Autodesk Inventor part; units mm, degrees
ref_plane "YZ Plane" through (0, 0, 0) normal (1, 0, 0) x (0, 1, 0)
ref_plane "XZ Plane" through (0, 0, 0) normal (0, 1, 0) x (-1, 0, 0)
ref_plane "XY Plane" through (0, 0, 0) normal (0, 0, 1) x (1, 0, 0)
sketch "Sketch1" plane through (0, 0, 0) normal (0, 1, 0) x (-1, 0, 0)
  line L0 (12.8, 0) -> (12.8, 32.2)
  line L1 (12.8, 16.1) -> (0, 16.1)
  line L2 (0, 0) -> (0, 32.2)
  line L3 (6.4, 27.2) -> (12.3, 27.2)
  line L4 (12.3, 27.2) -> (12.3, 5)
  line L5 (12.3, 5) -> (0.5, 5)
  line L6 (0.5, 5) -> (0.5, 27.2)
  line L7 (0.5, 27.2) -> (6.4, 27.2)
  line L8 (0, 0) -> (12.8, 0)
  circle A0 centre (6.4, 2.5) radius 0.5
  line L9 (0, 32.2) -> (12.8, 32.2)
  circle A1 centre (6.4, 29.7) radius 0.5
  line L10 (12.8, 32.2) -> (15.8, 32.2)
  line L11 (15.8, 32.2) -> (15.8, 0)
  line L12 (15.8, 0) -> (12.8, 0)
  line L13 (12.8, 0) -> (12.8, 32.2)
  point P0 (0, 0)
  dimension "d0" = 5.9
  dimension "d1" = 11.8
  dimension "d2" = 1
  dimension "d3" = 1
  dimension "d4" = 3
extrude "Extrusion1" add sketch "Sketch1" along normal blind 3 contours L8 L2 L1 L6 L5 L4 L0 | L0 L10 L11 L12 | L1 L4 L3 L7 L6 L2 L9 L0
sketch "Sketch2" plane through (0, 3, 0) normal (0, 1, 0) x (1, 0, 0)
  line L0 (-15.8, 0) -> (-15.8, -32.2)
  line L1 (0, 0) -> (-15.8, 0)
  line L2 (-15.8, -32.2) -> (-12.3, -32.2)
  line L3 (-12.3, -32.2) -> (-12.3, 0)
  line L4 (-12.3, 0) -> (-15.8, 0)
  line L5 (-15.8, 0) -> (-15.8, -32.2)
  dimension "d7" = 3.5
extrude "Extrusion2" add sketch "Sketch2" along normal blind 13
fillet "Fillet1" radius 2 1 edges at (-15.8, 0, 16.1)
sketch "Sketch3" plane through (-15.8, 16, 0) normal (-1, 0, 0) x (0, 0, 1)
  line L0 (32.2, -14) -> (32.2, 0)
  line L1 (32.2, -14) -> (0, -14)
  line L2 (32.2, 0) -> (51.999, 0) construction
  circle A0 centre (25.2, -7) radius 1.35
  line L3 (25.2, -7) -> (32.7, -7) construction
  circle A1 centre (17.7, -7) radius 0.65
  circle A2 centre (15.2, -7) radius 0.65
  circle A3 centre (12.7, -7) radius 0.65
  point P0 (0, -16)
  dimension "d12" = 2.7
  dimension "d17" = 1.3
  dimension "d18" = 1.3
  dimension "d19" = 1.3
extrude "Extrusion3" cut sketch "Sketch3" against normal blind 13
fillet "Fillet2" radius 2 4 edges at (-14.05, 16, 0) (-14.05, 16, 32.2) (0, 1.5, 32.2) (0, 1.5, 0)
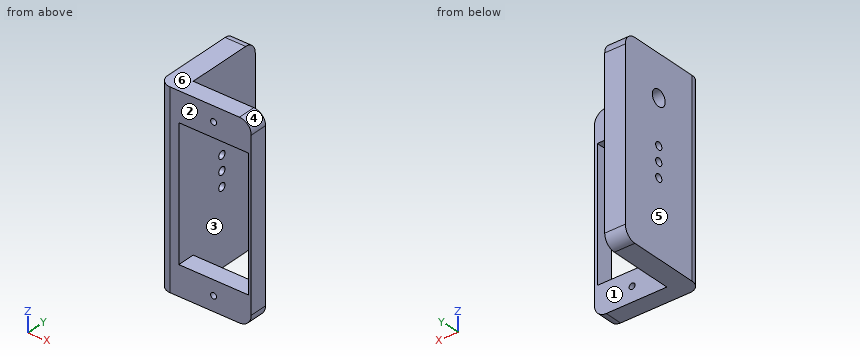
Geometry: final body of the model. Coordinates: model frame, mm. Face numbers are marked on the shaded views. A direction names the side the tool comes from. Give positions to 0.01 mm unless a question says otherwise; leave off trailing zeros. Loops run counter-clockwise (first coordinate to the right, second up) from the corner with the lowest first, then second, coordinate; pieces in that order, holes last. Notation, with made-up numbers: (-37, -33.75) -> (-1, -33.75) arc R27 cw to (-1, -14.75) -> close; hole circle Ø3 at (-0.75, 57). An arc over 180 degrees is marked (long way). Return JSON: item names as keys, results as strings.
Item 1: Mould query, pull axis X, two halves, no side actions, for the marked faces 3, 4, 5 and 6. Classes: released by +X, released by -X, zero draft, split by the parting line, or undercut.
Filled in:
{"face 3": "undercut", "face 4": "released by +X", "face 5": "released by -X", "face 6": "zero draft"}
Item 2: Pin query (flat end, axial travel): P1, Ø1.7, axis at y = 9, z = 17.7, coming from the +X side; P2, Ø6, axis at x = -11, z = 23.5, coming from the -Y side. Return the tip coordinate at first contact, or that it passes through.
Filled in:
{"P1": "x = -12.3", "P2": "y = 0"}
Item 3: Section D-D, the plane z = 29.7. Output: boundary loops of the cut face in (x, y).
Filled in:
{"outline": "(-15.8, 2) arc R2 ccw to (-13.8, 0) -> (-6.9, 0) -> (-6.9, 3) -> (-12.3, 3) -> (-12.3, 16) -> (-15.8, 16) -> close; (-5.9, 0) -> (0, 0) -> (0, 3) -> (-5.9, 3) -> close"}
Item 4: Section B-B, the plane z = 25.2. Output: boundary loops of the cut face in (x, y).
Filled in:
{"outline": "(-15.8, 2) arc R2 ccw to (-13.8, 0) -> (-12.3, 0) -> (-12.3, 7.65) -> (-15.8, 7.65) -> close; (-15.8, 10.35) -> (-12.3, 10.35) -> (-12.3, 16) -> (-15.8, 16) -> close; (-0.5, 0) -> (0, 0) -> (0, 3) -> (-0.5, 3) -> close"}
Item 5: Line query: line 1 (Y direction, x = -13.8, z = 25.2); line 2 (Z direction, x = -6.4, y = 0.75); line 3 (Z direction, x = -12.5, y = 8.5). Output: solid intervals per line, ascending.
Filled in:
{"line 1": "0 to 7.65, 10.35 to 16", "line 2": "0 to 2, 3 to 5, 27.2 to 29.2, 30.2 to 32.2", "line 3": "0 to 12.28, 13.12 to 14.78, 15.62 to 17.28, 18.12 to 23.95, 26.45 to 32.2"}
Item 6: Section C-C, the plane x = -12.75. Output: boundary loops of the cut face in (y, z).
Filled in:
{"outline": "(0, 0) -> (14, 0) arc R2 ccw to (16, 2) -> (16, 30.2) arc R2 ccw to (14, 32.2) -> (0, 32.2) -> close; hole circle Ø2.7 at (9, 25.2); hole circle Ø1.3 at (9, 12.7); hole circle Ø1.3 at (9, 15.2); hole circle Ø1.3 at (9, 17.7)"}
Item 7: Access query for the marked faces 1 and 2. Directions: +Z, -Z, +X, -X, +Y, -Y. A direction counts if a zero-diameter tool reaches every point of the face in a straight line with its end or side. Return the directions, or none.
Filled in:
{"face 1": "+Z, -Z, +X, +Y", "face 2": "+Z, -Z, +X, -X, -Y"}
Item 8: Section A-A, the plane x = -6.4. Output: boundary loops of the cut face in (y, z), plus the area to 3 significant figures.
Filled in:
{"outline": "(0, 0) -> (3, 0) -> (3, 2) -> (0, 2) -> close; (0, 3) -> (3, 3) -> (3, 5) -> (0, 5) -> close; (0, 27.2) -> (3, 27.2) -> (3, 29.2) -> (0, 29.2) -> close; (0, 30.2) -> (3, 30.2) -> (3, 32.2) -> (0, 32.2) -> close", "area": "24.0 mm^2"}
